from build123d import *

# Parameters (mm, degrees)
EXTRUDE_1_DEPTH     = 7.58
SKETCH_2_R          = 1
CUT_EXTRUDE_1_DEPTH = 10


with BuildPart() as part:
    # 草图1 → 凸台-拉伸1 (new body)
    with BuildSketch(Plane.XY):
        with BuildLine():
            Line((-77.371685393, 43.405828583), (69.028314607, 43.405828583))
            ThreePointArc((69.028314607, 43.405828583), (74.685168856, 41.062682833), (77.028314607, 35.405828583))
            Line((77.028314607, 35.405828583), (77.028314607, -22.794171417))
            ThreePointArc((77.028314607, -22.794171417), (74.685168856, -28.451025666), (69.028314607, -30.794171417))
            Line((69.028314607, -30.794171417), (-77.371685393, -30.794171417))
            ThreePointArc((-77.371685393, -30.794171417), (-83.028539643, -28.451025666), (-85.371685393, -22.794171417))
            Line((-85.371685393, -22.794171417), (-85.371685393, 35.405828583))
            ThreePointArc((-85.371685393, 35.405828583), (-83.028539643, 41.062682833), (-77.371685393, 43.405828583))
        make_face()
    extrude(amount=EXTRUDE_1_DEPTH)

    # 草图2 → 切除-拉伸1 (cut)
    with BuildSketch(Plane(origin=(77.028314607, 0, 0), x_dir=(0, 0, -1), z_dir=(1, 0, 0))):
        with Locations((-3.91637094, 31.096940443)):
            Circle(SKETCH_2_R)
        with Locations((-3.91637094, 28.096940443)):
            Circle(SKETCH_2_R)
        with Locations((-3.91637094, 25.096940443)):
            Circle(SKETCH_2_R)
        with Locations((-3.91637094, 22.096940443)):
            Circle(SKETCH_2_R)
        with Locations((-3.888231768, 19.096940443)):
            Circle(SKETCH_2_R)
        with BuildLine():
            Line((-1.869713351, 11.20207357), (-1.843333719, -0.047567419))
            ThreePointArc((-1.843333719, -0.047567419), (-3.838638371, -2.05225177), (-5.843322722, -0.056947118))
            Line((-5.843322722, -0.056947118), (-5.869702354, 11.192693871))
            ThreePointArc((-5.869702354, 11.192693871), (-3.874397702, 13.197378222), (-1.869713351, 11.20207357))
        make_face()
        with BuildLine():
            Line((-1.811351016, -13.686647662), (-1.799774442, -18.623498185))
            ThreePointArc((-1.799774442, -18.623498185), (-3.795079095, -20.628182535), (-5.799763445, -18.632877883))
            Line((-5.799763445, -18.632877883), (-5.811340019, -13.69602736))
            ThreePointArc((-5.811340019, -13.69602736), (-3.816035367, -11.69134301), (-1.811351016, -13.686647662))
        make_face()
    extrude(amount=-CUT_EXTRUDE_1_DEPTH, mode=Mode.SUBTRACT)


solid = part.part
Could you check a few things on this model? Use its own coordinates, in mm. A direction names the side the tool comes from. Round coordinates to 2 decimals unless told otherwise and drop trailing zeros. Write each loop counter-clockwise with the first axis right and the second up, starting at its lowest first coordinate (ties: lowest second). Pieces come first, ordered by that corner, then holes. Notation, with made-up numbers: (56.5, -11) - (112.5, -11) arc R23 ccw to (112.5, 2) - close; hole circle Ø4 at (21, 78.5). An arc over 180 degrees is marked (long way). Put each result on its own line as item: value. Start each with the question number.
(1) Thinking about a two-plate mould opening in Z: for faces 1 (the cylindrical face through (-82.97, -28.51, 3.74)), 2 (the flat face through (67.028, 6, 4)), 3 (the flat face through (-3, 7, 0)), which applies, released by +Z, released by -Z, zero draft, split by the parting line, or undercut?
(2) I need wall thicknesses on probe 1 along X at (y, z) = (0, 5); probe 2 along X at (y, z) = (-24, 7.25). Which ranges of each line are inside material? Lowest first, please.
(3) Will this pin go through, and if not, where does the flat tip stop? pin 1 (0.6 mm diameter, centred on y = 19, z = 3.5, fed in from +X).
(4) For faces 4 (the cylindrical face through (72.1, -2.05, 3.79)), 5 (the flat face through (-85.372, 6, 4)), which set-ups out of +Z, -Z, +X, -X, +Y, -Y let a thin tool reach every point of the face, with its end or its side?
(5) I want a section at A-A, the plane y = -15.5. Please give me the cut outline in (x, z).
Here are the results:
1. face 1: zero draft
1. face 2: undercut
1. face 3: released by -Z
2. probe 1: x = -85.37 to 67.03
2. probe 2: x = -85.28 to 76.94
3. pin 1: stops at x = 67.03
4. face 4: +X
4. face 5: +Z, -Z, -X, +Y, -Y
5. outline: (-85.37, 0) - (77.03, 0) - (77.03, 1.81) - (67.03, 1.81) - (67.03, 5.81) - (77.03, 5.81) - (77.03, 7.58) - (-85.37, 7.58) - close
